Part model, mm, in its own coordinate system. Face numbers are marked on the shaded views. A direction names the side the tool comes from. Round coordinates to 2 decimals unless told otherwise and drop trailing zeros. Write each loop counter-clockwise with the first axis right and the second up, starting at its lowest first coordinate (ties: lowest second). Pieces come first, ordered by that corner, then holes.
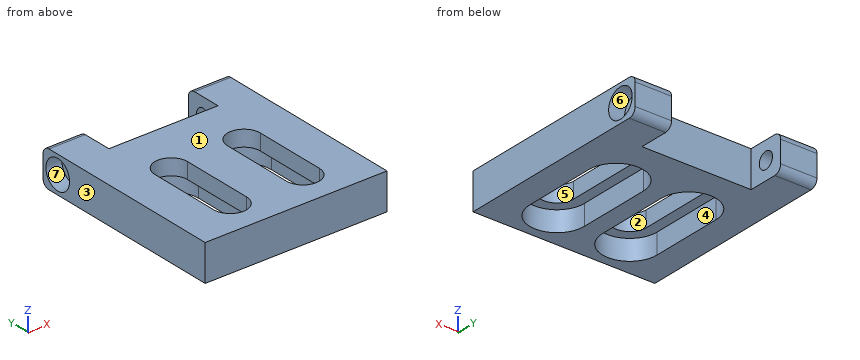
from build123d import *

# Parameters (mm, degrees)
SKETCH1_W           = 50
SKETCH1_H           = 55
BOSS_EXTRUDE3_DEPTH = 10
SKETCH2_W           = 30
SKETCH2_H           = 10
CUT_EXTRUDE2_DEPTH  = 10
CUT_EXTRUDE3_DEPTH  = 5.6
FILLET1_R           = 2


with BuildPart() as part:
    # Sketch1 → Boss-Extrude3 (new body)
    with BuildSketch(Plane.XY):
        Rectangle(SKETCH1_W, SKETCH1_H)
        with BuildLine():
            Line((-5.5, 2.5), (-5.5, -17.5))
            ThreePointArc((-5.5, -17.5), (-10, -22), (-14.5, -17.5))
            Line((-14.5, -17.5), (-14.5, 2.5))
            ThreePointArc((-14.5, 2.5), (-10, 7), (-5.5, 2.5))
        make_face(mode=Mode.SUBTRACT)
        with BuildLine():
            Line((5.5, 2.5), (5.5, -17.5))
            ThreePointArc((5.5, -17.5), (10, -22), (14.5, -17.5))
            Line((14.5, -17.5), (14.5, 2.5))
            ThreePointArc((14.5, 2.5), (10, 7), (5.5, 2.5))
        make_face(mode=Mode.SUBTRACT)
    extrude(amount=BOSS_EXTRUDE3_DEPTH)

    # Sketch2 → Cut-Extrude2 (cut)
    with BuildSketch(Plane(origin=(0, 0, 0), x_dir=(-1, 0, 0), z_dir=(0, 0, -1))):
        with Locations((0, 22.5)):
            Rectangle(SKETCH2_W, SKETCH2_H)
    extrude(amount=-CUT_EXTRUDE2_DEPTH, mode=Mode.SUBTRACT)

    # Sketch6 → CBORE for M4 Hex Socket Head Cap Screw1 (revolve, cut)
    with BuildSketch(Plane(origin=(25, 22.5, 5), x_dir=(0, 0, -1), z_dir=(0, 1, 0))):
        Polygon((0, 0), (0, 15.351936393), (2.25, 14), (2.25, 4.4), (4, 4.4), (4, 0), align=None)
    cbore_for_m4_hex_socket_head_cap_screw1 = revolve(axis=Axis((31.35, 22.5, 5), (-1, 0, 0)), mode=Mode.SUBTRACT)

    # Mirror1: CBORE for M4 Hex Socket Head Cap Screw1 across plane
    add(cbore_for_m4_hex_socket_head_cap_screw1.mirror(Plane(origin=(0, 0, 0), x_dir=(0, 0, 1), z_dir=(1, 0, 0))), mode=Mode.SUBTRACT)

    # Sketch7 → Cut-Extrude3 (cut)
    with BuildSketch(Plane(origin=(0, 0, 0), x_dir=(-1, 0, 0), z_dir=(0, 0, -1))):
        with BuildLine():
            Line((-2.5, 2.5), (-2.5, -17.5))
            ThreePointArc((-2.5, -17.5), (-10, -25), (-17.5, -17.5))
            Line((-17.5, -17.5), (-17.5, 2.5))
            ThreePointArc((-17.5, 2.5), (-10, 10), (-2.5, 2.5))
        make_face()
        with BuildLine():
            Line((2.5, 2.5), (2.5, -17.5))
            ThreePointArc((2.5, -17.5), (10, -25), (17.5, -17.5))
            Line((17.5, -17.5), (17.5, 2.5))
            ThreePointArc((17.5, 2.5), (10, 10), (2.5, 2.5))
        make_face()
    extrude(amount=-CUT_EXTRUDE3_DEPTH, mode=Mode.SUBTRACT)

    # Fillet1
    fillet1_edges = [part.edges().sort_by_distance(p)[0] for p in [
        (-20, 27.5, 0),
        (-20, 27.5, 10),
        (20, 27.5, 0),
        (20, 27.5, 10),
    ]]
    fillet(fillet1_edges, radius=FILLET1_R)


solid = part.part
Q1. Saw through at C-C, the plane x = -20. Write the cut outline in (y, z), and give its area (3 significant figures).
Q2. Saw through at A-A, the plane x = -10. Write the cut outline in (y, z).
Q3. Tool access for the marked faces 5, 6 and 7: list every direction of +Z, -Z, +X, -X, +Y, -Y with a clear straight run to the whole face (end or side of a thin tool).
Q4. Saw through at D-D, the plane y = -7. Write the cut outline in (x, z).
Q5. Drop flat-ended pins along their axis: P1, Ø3, axis at x = 7, z = 6, coming from the +Y side; P2, Ø2.5, axis at y = 22.5, z = 5, coming from the -X side. Give the stop position or say it passes through.
Q6. Saw through at B-B, the plane y = 22.5. Write the cut outline in (x, z), and give its area (3 significant figures).
Q7. Two-plate mould, pull along X, no slides. Class the marked faces 1, 2, 3 and 4: released by +X, released by -X, zero draft, split by the parting line, or undercut.
Q8. Wall check: line 1 (X direction, y = -15, z = 9); line 2 (Y direction, x = -23, z = 5); line 3 (Y direction, x = -16, z = 2.5). Give the ranges that are in metal, low to high.
Computed:
1. outline: (-27.5, 0) - (25.5, 0) arc R2 ccw to (27.5, 2) - (27.5, 8) arc R2 ccw to (25.5, 10) - (-27.5, 10) - close; hole circle Ø4.5 at (22.5, 5)
1. area: 532 mm2
2. outline: (-27.5, 0) - (-25, 0) - (-25, 5.6) - (-22, 5.6) - (-22, 10) - (-27.5, 10) - close; (7, 5.6) - (10, 5.6) - (10, 0) - (17.5, 0) - (17.5, 10) - (7, 10) - close
3. face 5: +Z, -Z
3. face 6: +X
3. face 7: -X
4. outline: (-25, 0) - (-17.5, 0) - (-17.5, 5.6) - (-14.5, 5.6) - (-14.5, 10) - (-25, 10) - close; (-5.5, 5.6) - (-2.5, 5.6) - (-2.5, 0) - (2.5, 0) - (2.5, 5.6) - (5.5, 5.6) - (5.5, 10) - (-5.5, 10) - close; (14.5, 5.6) - (17.5, 5.6) - (17.5, 0) - (25, 0) - (25, 10) - (14.5, 10) - close
5. P1: stops at y = 17.5
5. P2: passes through
6. outline: (-25, 0) - (-15, 0) - (-15, 2.75) - (-20.6, 2.75) - (-20.6, 1) - (-25, 1) - close; (-25, 9) - (-20.6, 9) - (-20.6, 7.25) - (-15, 7.25) - (-15, 10) - (-25, 10) - close; (15, 0) - (25, 0) - (25, 1) - (20.6, 1) - (20.6, 2.75) - (15, 2.75) - close; (15, 7.25) - (20.6, 7.25) - (20.6, 9) - (25, 9) - (25, 10) - (15, 10) - close
6. area: 79.2 mm2
7. face 1: zero draft
7. face 2: undercut
7. face 3: released by -X
7. face 4: undercut
8. line 1: x = -25 to -14.5, -5.5 to 5.5, 14.5 to 25
8. line 2: y = -27.5 to 18.5, 26.5 to 27.5
8. line 3: y = -27.5 to -22, 7 to 27.5
